from build123d import *

# Parameters (mm, degrees)
SKETCH1_W           = 205
SKETCH1_H           = 42
BOSS_EXTRUDE1_DEPTH = 6.35
SKETCH4_R           = 11
CUT_EXTRUDE3_DEPTH  = 7.35
CHAMFER1_SIZE       = 5
SKETCH9_R           = 11
CUT_EXTRUDE8_DEPTH  = 7.35
SKETCH14_R          = 11
SKETCH14_R_2        = 2.413
CUT_EXTRUDE10_DEPTH = 10


with BuildPart() as part:
    # Sketch1 → Boss-Extrude1 (new body)
    with BuildSketch(Plane.XY):
        Rectangle(SKETCH1_W, SKETCH1_H)
    extrude(amount=BOSS_EXTRUDE1_DEPTH)

    # Sketch4 → Cut-Extrude3 (cut, through all)
    with BuildSketch(Plane.XY.offset(6.35)):
        with Locations((-78.5, 0)):
            Circle(SKETCH4_R)
    extrude(amount=-CUT_EXTRUDE3_DEPTH, mode=Mode.SUBTRACT)

    # Chamfer1
    chamfer1_edges = [part.edges().sort_by_distance(p)[0] for p in [
        (102.5, -21, 3.175),
        (-102.5, -21, 3.175),
        (-102.5, 21, 3.175),
        (102.5, 21, 3.175),
    ]]
    chamfer(chamfer1_edges, length=CHAMFER1_SIZE)

    # Sketch9 → Cut-Extrude8 (cut, through all)
    with BuildSketch(Plane.XY.offset(6.35)):
        with Locations((82.5, 0)):
            Circle(SKETCH9_R)
    extrude(amount=-CUT_EXTRUDE8_DEPTH, mode=Mode.SUBTRACT)

    # Sketch14 → Cut-Extrude10 (cut)
    with BuildSketch(Plane.XY.offset(6.35)):
        Polygon((-47.5, -16), (-47.5, 16), (-42.5, 21), (-97.5, 21), (-102.5, 16), (-102.5, -16), (-97.5, -21), (-42.5, -21), align=None)
        with Locations((-78.5, 0)):
            Circle(SKETCH14_R, mode=Mode.SUBTRACT)
        with Locations((-27.5, 10)):
            Circle(SKETCH14_R_2)
        with Locations((-27.5, -10)):
            Circle(SKETCH14_R_2)
        with Locations((-12.5, -10)):
            Circle(SKETCH14_R_2)
        with Locations((-12.5, 10)):
            Circle(SKETCH14_R_2)
        with Locations((17.5, 10)):
            Circle(SKETCH14_R_2)
        with Locations((2.5, -10)):
            Circle(SKETCH14_R_2)
        with Locations((17.5, -10)):
            Circle(SKETCH14_R_2)
        with Locations((2.5, 10)):
            Circle(SKETCH14_R_2)
    extrude(amount=-CUT_EXTRUDE10_DEPTH, mode=Mode.SUBTRACT)


solid = part.part
Could you check a few things on this model? Use its own coordinates, in mm. Give positions to 0.01 mm unless a question says otherwise; leave off trailing zeros. Order: outer loops, then holes, each group sorted by start corner. A loop starts at its lowest first (then second) coordinate and runs counter-clockwise, first axis right, second up. Notation, with made-up numbers: (47, 64.25) -> (64, 64.25) arc R23 ccw to (64, 83.25) -> close; hole circle Ø5 at (88.25, -23.5). An arc over 180 degrees is marked (long way). Answer in a Markdown table with one row per item. Add a question column.
Item 1: Imagine slicing it at B-B (x = -12.5). List the corners of the cut face in (y, z) for me, and give its area (3 significant figures).
Item 2: Imagine slicing it at D-D (x = 82.5). List the corners of the cut face in (y, z) for me, and give its area (3 significant figures).
Item 3: Imagine slicing it at C-C (y = 3.5). List the corners of the cut face in (x, z) for me.
Item 4: Imagine slicing it at A-A (z = 1.25). Count the separate pieces of the cut face and the enclosed holes in it, and give its area (3 significant figures).
Item 5: We'd pull the mould along X, two halves only. Please class faces 1 (the cylindrical face through (-14.28, -8.37, 3.22)), 2 (the flat face through (102.5, 0, 3)), 3 (the flat face through (27, -21, 3)): pulls with the +X half, pulls with the -X half, needs draft (parallel to the pull), parting line crosses it, or undercut.
Item 6: Please list where these lines run through material, in increasing order: probe 1 along Y at (x, z) = (-12.5, 4.5); probe 2 along X at (y, z) = (9, 4.75); probe 3 along Y at (x, z) = (1, 0.5).
Result:
| question | item | result |
|---|---|---|
| 1 | outline | (-21, 0) -> (-12.41, 0) -> (-12.41, 6.35) -> (-21, 6.35) -> close; (-7.59, 0) -> (7.59, 0) -> (7.59, 6.35) -> (-7.59, 6.35) -> close; (12.41, 0) -> (21, 0) -> (21, 6.35) -> (12.41, 6.35) -> close |
| 1 | area | 205 mm2 |
| 2 | outline | (-21, 0) -> (-11, 0) -> (-11, 6.35) -> (-21, 6.35) -> close; (11, 0) -> (21, 0) -> (21, 6.35) -> (11, 6.35) -> close |
| 2 | area | 127 mm2 |
| 3 | outline | (-47.5, 0) -> (72.07, 0) -> (72.07, 6.35) -> (-47.5, 6.35) -> close; (92.93, 0) -> (102.5, 0) -> (102.5, 6.35) -> (92.93, 6.35) -> close |
| 4 | separate pieces | 1 |
| 4 | enclosed holes | 9 |
| 4 | area | 5,720 mm2 |
| 5 | face 1 | undercut |
| 5 | face 2 | pulls with the +X half |
| 5 | face 3 | needs draft |
| 6 | probe 1 | -21 to -12.41, -7.59 to 7.59, 12.41 to 21 |
| 6 | probe 2 | -47.5 to -29.7, -25.3 to -14.7, -10.3 to 0.3, 4.7 to 15.3, 19.7 to 76.18, 88.82 to 102.5 |
| 6 | probe 3 | -21 to -11.89, -8.11 to 8.11, 11.89 to 21 |
